Source: CAD feature listing. Evaluate the final solid. Frame: model axes, mm. Give positions to 0.01 mm unless a question says otherwise; leave off trailing zeros. Write each loop counter-clockwise with the first axis right and the second up, starting at its lowest first coordinate (ties: lowest second). Pieces come first, ordered by that corner, then holes. Notation, with made-up numbers: (60, 49) -> (87, 49) arc R10 cw to (87, 68) -> close; hole circle Ø6 at (1.5, 55). An arc over 180 degrees is marked (long way). Use one line per item in the form item = value. Start each with the question number.
(1) First-contact query: P1, Ø10, axis at x = -6.5, y = 7, coming from the -Z side; P2, Ø4, axis at x = 5, y = 5.5, coming from the -Z side; P3, Ø5, axis at x = 1, z = 8, coming from the +Y side; P4, Ø1.5, axis at x = -1.5, y = -1.5, coming from the -Z side. Flat tips, straight axial feed; report the tip coordinate or a pass-through.
(2) Cut plane D-D, the plane z = 10. Output: boundary loops of the cut face in (x, y).
(3) Cut plane C-C, the plane y = 5. Output: boundary loops of the cut face in (x, z).
(4) Material intervals for line 1 along Z through (x, y) = (0, 1.5); line 2 along Z through (x, y) = (0, -1), sorted ascending. Write a range as from..to.
(5) Cut plane A-A, the plane z = 0. Output: boundary loops of the cut face in (x, y).
(6) Cut plane B-B, the plane x = 0. Output: boundary loops of the cut face in (y, z).
(7) Draft query along Z for faces 1 (the face through (1, -0.28, -0.32)), 2 (the face through (3, -16, 0)), 3 (the face through (-0.54, 7.4, 2.44)). Return one class per face: pulls with the +Z half, pulls with the -Z half, needs draft (parallel to the pull), parting line crosses it, or undercut.
from build123d import *

# Parameters (mm, degrees)
SKETCH_R     = 14.5
PAD_DEPTH    = 16
SKETCH001_R  = 2.5
PAD001_DEPTH = 15
SKETCH002_R  = 1.05
POCKET_DEPTH = 31.001


with BuildPart() as part:
    # Sketch → Pad (new body)
    with BuildSketch(Plane.XZ):
        Circle(SKETCH_R)
    extrude(amount=PAD_DEPTH)

    # Sketch001 (on Face2 of Pad) → Pad001 (join)
    with BuildSketch(Plane(origin=(0, 0, 0), x_dir=(1, 0, 0), z_dir=(0, 1, 0))):
        Circle(SKETCH001_R)
    extrude(amount=PAD001_DEPTH)

    # Sketch002 (on Face5 of Pad001) → Pocket (cut, through all)
    with BuildSketch(Plane(origin=(0, 15, 0), x_dir=(1, 0, 0), z_dir=(0, 1, 0))):
        Circle(SKETCH002_R)
    extrude(amount=-POCKET_DEPTH, mode=Mode.SUBTRACT)


solid = part.part
Geometry says:
q1.P1 = -2
q1.P2 = through
q1.P3 = 0
q1.P4 = -14.48
q2.outline = (-10.5, -16) -> (10.5, -16) -> (10.5, 0) -> (-10.5, 0) -> close
q3.outline = circle Ø5 at (0, 0); hole circle Ø2.1 at (0, 0)
q4.line_1 = -2.5..-1.05, 1.05..2.5
q4.line_2 = -14.5..-1.05, 1.05..14.5
q5.outline = (-14.5, -16) -> (-1.05, -16) -> (-1.05, 15) -> (-2.5, 15) -> (-2.5, 0) -> (-14.5, 0) -> close; (1.05, -16) -> (14.5, -16) -> (14.5, 0) -> (2.5, 0) -> (2.5, 15) -> (1.05, 15) -> close
q6.outline = (-16, -14.5) -> (0, -14.5) -> (0, -2.5) -> (15, -2.5) -> (15, -1.05) -> (-16, -1.05) -> close; (-16, 1.05) -> (15, 1.05) -> (15, 2.5) -> (0, 2.5) -> (0, 14.5) -> (-16, 14.5) -> close
q7.face_1 = undercut
q7.face_2 = needs draft
q7.face_3 = parting line crosses it
